Source: CAD feature listing. Evaluate the final solid. Frame: model axes, mm. A direction names the side the tool comes from. Give positions to 0.01 mm unless a question says otherwise; leave off trailing zeros. Order: outer loops, then holes, each group sorted by start corner. A loop starts at its lowest first (then second) coordinate and runs counter-clockwise, first axis right, second up. Notation, with made-up numbers: (-19.5, 83) -> (23.5, 83) arc R20 ccw to (23.5, 102) -> close; hole circle Ø1 at (43.25, -38.75). An arc over 180 degrees is marked (long way). Use one line per item in the form item = value. Start each with the question number.
from build123d import *

# Parameters (mm, degrees)
F1_DEPTH  = 4.318
F2_DEPTH  = 1.778
F3_SIZE   = 0.508
F4_SIZE   = 0.508
F5_SIZE   = 0.508
F6_DEPTH  = 2.54
F7_DEPTH  = 2.54
F8_SIZE   = 2.53999
F9_SIZE   = 2.53999
F11_DEPTH = 0.254
F12_DEPTH = 0.254


# Not quite as in the source:
# - a fillet or chamfer is up to 0.001 mm smaller than in the source, because OpenCascade refuses the exact size
# - a feature names something its author has since deleted; it is built from what else it names


with BuildPart() as f1:
    # F0 (on Top) → F1 (new body)
    with BuildSketch(Plane.XY):
        Polygon((-6.35, 0), (0, 0), (0, 3.81), align=None)
        Polygon((0, 3.81), (0, 0), (6.35, 0), align=None)
        Polygon((6.35, 0), (0, 0), (0, -3.81), align=None)
        Polygon((0, -3.81), (0, 0), (-6.35, 0), align=None)
    extrude(amount=F1_DEPTH)

    # F5
    f5_edges = [f1.edges().sort_by_distance(p)[0] for p in [
        (-3.175, -1.905, 4.318),
        (3.175, -1.905, 4.318),
        (3.175, 1.905, 4.318),
        (-3.175, 1.905, 4.318),
    ]]
    chamfer(f5_edges, length=F5_SIZE)

    # F7 (add): a face of the model
    f7_faces = [f1.faces().sort_by_distance(p)[0] for p in [
        (0, 0, 4.318),
    ]]
    extrude(f7_faces, amount=F7_DEPTH)

    # F8 (size 2.54 in the source; OpenCascade refuses exactly that, so slightly less here)
    f8_edges = [f1.edges().sort_by_distance(p)[0] for p in [
        (-2.681313, -1.608788, 6.858),
        (-2.681313, 1.608788, 6.858),
        (2.681313, -1.608788, 6.858),
        (2.681313, 1.608788, 6.858),
    ]]
    chamfer(f8_edges, length=F8_SIZE)


with BuildPart() as f2:
    # F0 (on Top) → F2 (new body)
    with BuildSketch(Plane.XY):
        Polygon((6.35, 0), (0, 0), (0, -3.81), align=None)
        Polygon((0, -3.81), (0, 0), (-6.35, 0), align=None)
        Polygon((0, 3.81), (0, 0), (6.35, 0), align=None)
        Polygon((-6.35, 0), (0, 0), (0, 3.81), align=None)
    extrude(amount=-F2_DEPTH)

    # F3
    f3_edges = [f2.edges().sort_by_distance(p)[0] for p in [
        (3.175, 1.905, -1.778),
        (3.175, -1.905, -1.778),
    ]]
    chamfer(f3_edges, length=F3_SIZE)

    # F4
    f4_edges = [f2.edges().sort_by_distance(p)[0] for p in [
        (-3.421844, 1.756894, -1.778),
        (-3.421844, -1.756894, -1.778),
    ]]
    chamfer(f4_edges, length=F4_SIZE)

    # F6 (add): a face of the model
    f6_faces = [f2.faces().sort_by_distance(p)[0] for p in [
        (0, 0, -1.778),
    ]]
    extrude(f6_faces, amount=F6_DEPTH)

    # F9 (size 2.54 in the source; OpenCascade refuses exactly that, so slightly less here)
    f9_edges = [f2.edges().sort_by_distance(p)[0] for p in [
        (2.681313, 1.608788, -4.318),
        (-2.681313, 1.608788, -4.318),
        (2.681313, -1.608788, -4.318),
        (-2.681313, -1.608788, -4.318),
    ]]
    chamfer(f9_edges, length=F9_SIZE)

    # F10: union F1
    add(f1.part)

    # F11 (cut): faces of the model
    f11_faces = [f2.faces().sort_by_distance(p)[0] for p in [
        (3.175, 1.905, 1.27),
        (-3.175, 1.905, 1.27),
        (-3.175, -1.905, 1.27),
        (3.175, -1.905, 1.27),
    ]]
    extrude(f11_faces, amount=-F11_DEPTH, dir=(0.5144957554, 0.8574929257, 0), mode=Mode.SUBTRACT)

    # F12 (cut): faces of the model
    f12_faces = [f2.faces().sort_by_distance(p)[0] for p in [
        (-3.1169191458, -1.9398485125, 1.27),
        (3.0515781849, -1.9790530891, 1.27),
    ]]
    extrude(f12_faces, amount=-F12_DEPTH, dir=(-0.5144957554, -0.8574929257, 0), mode=Mode.SUBTRACT)


solid = f2.part
1) Cut plane C-C, the plane z = 0.5. Return the cut outline in (x, y).
2) Material intervals for probe 1 along Z at (x, y) = (0.75, -3); probe 2 along Y at (x, z) = (1.5, 2.5); probe 3 along X at (y, z) = (-2.5, -0.5), sorted ascending.
3) Cut plane D-D, the plane z = -3.25. Return the cut outline in (x, y), plus the area to 3 significant figures.
4) Reachability of faces 1 (the face through (-3.02, 1.86, 1.23)), 2 (the face through (-3, 1.71, 4.07)), 3 (the face through (2.97, 1.73, 1.23)) from +Z, -Z, +X, -X, +Y, -Y: full face, straight path, thin tool, end or side. Return the list, or none.
5) Draft query along Z for faces 4 (the face through (3.02, -1.86, 1.23)), 5 (the face through (-3, 1.72, -1.52)), 6 (the face through (3.087, 1.657, 4.068)). Return one class per face: +Z half, -Z half, draft (parallel to the pull), parting line (faces both ways), or undercut.
6) Pin query (flat end, axial travel): pin 1 (6 mm diameter, centred on x = -3, z = 5, fed in from -Y); pin 2 (4 mm diameter, centred on x = -3.5, y = -3, fed in from +Z). Return the tip coordinate at first contact, or that it passes through.
Output values:
q1.outline = (-5.99, 0.08) -> (0.13, -3.59) -> (5.99, -0.08) -> (-0.13, 3.59) -> close
q2.probe_1 = -1.58 to 4.12
q2.probe_2 = -2.77 to 2.61
q2.probe_3 = -1.69 to 1.95
q3.outline = (-2.5, 0) -> (0, -1.5) -> (2.5, 0) -> (0, 1.5) -> close
q3.area = 7.51 mm^2
q4.face_1 = -X, +Y
q4.face_2 = +Z, -X, +Y
q4.face_3 = +X, +Y
q5.face_4 = undercut
q5.face_5 = -Z half
q5.face_6 = +Z half
q6.pin_1 = -3.66
q6.pin_2 = 4.7
